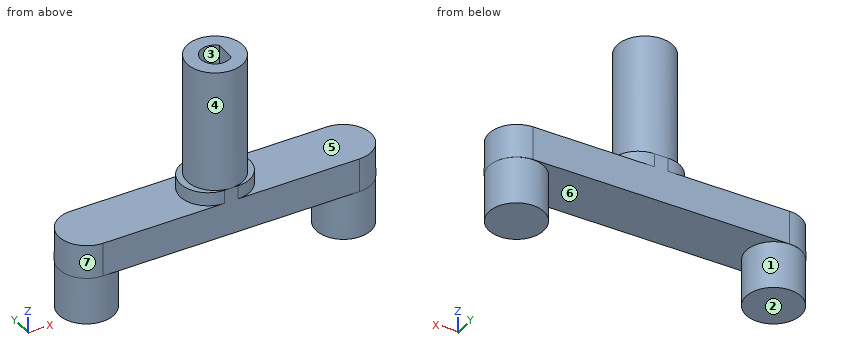
```python
from build123d import *

# Parameters (mm, degrees)
PAD007_DEPTH    = 5
PAD008_DEPTH    = 2
SKETCH010_R     = 4.05
PAD009_DEPTH    = 7
SKETCH012_R     = 4.1
PAD011_DEPTH    = 18
POCKET002_DEPTH = 10


with BuildPart() as part:
    # Sketch007 → Pad007 (new body)
    with BuildSketch(Plane.XY):
        with BuildLine():
            ThreePointArc((-18.65, 4.1), (-22.75, 0), (-18.65, -4.1))
            Line((-18.65, -4.1), (18.65, -4.1))
            ThreePointArc((18.65, -4.1), (22.75, 0), (18.65, 4.1))
            Line((-18.65, 4.1), (18.65, 4.1))
        make_face()
    extrude(amount=PAD007_DEPTH)

    # Sketch008 (on Face6 of Pad007) → Pad008 (join)
    with BuildSketch(Plane.XY.offset(5)):
        with BuildLine():
            ThreePointArc((-1, 4.1), (-5.1, 0), (-1, -4.1))
            Line((-1, -4.1), (1, -4.1))
            ThreePointArc((1, -4.1), (5.1, 0), (1, 4.1))
            Line((-1, 4.1), (1, 4.1))
        make_face()
    extrude(amount=PAD008_DEPTH)

    # Sketch010 → Pad009 (join)
    with BuildSketch(Plane(origin=(0, 0, 0), x_dir=(1, 0, 0), z_dir=(0, 0, -1))):
        with Locations((-18.7, 0)):
            Circle(SKETCH010_R)
        with Locations((18.7, 0)):
            Circle(SKETCH010_R)
    extrude(amount=PAD009_DEPTH)

    # Sketch012 (on Face8 of Pad008) → Pad011 (join)
    with BuildSketch(Plane.XY.offset(7)):
        Circle(SKETCH012_R)
    extrude(amount=PAD011_DEPTH)

    # Sketch009 (on Face17 of Pad011) → Pocket002 (cut)
    with BuildSketch(Plane.XY.offset(25)):
        with BuildLine():
            Line((1.5, 1.469694), (1.5, -1.469694))
            ThreePointArc((1.5, 1.469694), (-2.1, 0), (1.5, -1.469694))
        make_face()
    extrude(amount=-POCKET002_DEPTH, mode=Mode.SUBTRACT)


solid = part.part
```
CAD build for the part. Positions are in the model's coordinates, mm. Face numbers are marked on the shaded views. A direction names the side the tool comes from. Round coordinates to 2 decimals unless told otherwise and drop trailing zeros. Loops run counter-clockwise (first coordinate to the right, second up) from the corner with the lowest first, then second, coordinate; pieces in that order, holes last. Notation, with made-up numbers: (84, 3.5) - (104, 3.5) arc R20 cw to (104, 21.5) - close; hole circle Ø8 at (-14.5, 14). An arc over 180 degrees is marked (long way). Return JSON: item names as keys, results as strings. Group by question number.
Q1. Band-saw the part on D-D on z = 19. Give the cut face in (x, y), plus the area to 3 significant figures.
Q2. Two-plate mould, pull along X, no slides. Class the marked faces 4, 5, 6 and 7: +X half, -X half, draft (parallel to the pull), parting line (faces both ways), or undercut.
Q3. Tool access for the marked faces 1, 2 and 3: list every direction of +Z, -Z, +X, -X, +Y, -Y with a clear straight run to the whole face (end or side of a thin tool).
Q4. Flat gauge pins, fed straight in: pin 1 Ø2.5 at (x, y) = (16.5, -1) entering from +Z; pin 2 Ø3 at (x, y) = (-1, 0.5) entering from +Z; pin 3 Ø3 at (y, z) = (0.5, 18.5) entering from -X; pin 4 Ø1 at (x, y) = (-2.5, -1.5) entering from -Z. Where does each tip first touch, or does it go through?
Q5. Band-saw the part on B-B on z = 1. Give the cut face in (x, y), plus the area to 3 significant figures.
Q6. Drill centre lines: line 1 along X through (y, z) = (0, 20); line 2 along Y through (x, z) = (0, 21); line 3 along X through (y, z) = (-0.25, 4). Where is each one in solid material? Low to high. Write a range as [from, to].
Solutions:
{
 "1": {"outline": "circle Ø8.2 at (0, 0); hole (1.5, -1.47) - (1.5, 1.47) arc R2.1 ccw (long way) to start", "area": "40.2 mm^2"},
 "2": {"face 4": "parting line", "face 5": "draft", "face 6": "undercut", "face 7": "-X half"},
 "3": {"face 1": "-Z", "face 2": "-Z, +X, -X, +Y, -Y", "face 3": "+Z"},
 "4": {"pin 1": "stops at z = 5", "pin 2": "stops at z = 25", "pin 3": "stops at x = -4.1", "pin 4": "stops at z = 0"},
 "5": {"outline": "(-18.65, -4.1) - (18.65, -4.1) arc R4.1 ccw to (18.65, 4.1) - (-18.65, 4.1) arc R4.1 ccw to start", "area": "359 mm^2"},
 "6": {"line 1": "x = [-4.1, -2.1], [1.5, 4.1]", "line 2": "y = [-4.1, -2.1], [2.1, 4.1]", "line 3": "x = [-22.74, 22.74]"}
}
